```python
from build123d import *

# Parameters (mm, degrees)
SKETCH1_W            = 308.08168
SKETCH1_H            = 3.175
BOSS_EXTRUDE1_DEPTH  = 267.83
SKETCH3_W            = 267.83
SKETCH3_H            = 3.175
BOSS_EXTRUDE3_DEPTH  = 3.175
SKETCH4_W            = 50.8889
SKETCH4_H            = 3.175
BOSS_EXTRUDE4_DEPTH  = 267.83
CUT_EXTRUDE1_DEPTH   = 340.191055801
SKETCH17_W           = 267.83
SKETCH17_H           = 3.175
BOSS_EXTRUDE5_DEPTH  = 3.175
CUT_EXTRUDE3_DEPTH   = 340.191055801
SKETCH25_R           = 3.175
CUT_EXTRUDE8_DEPTH   = 3.175
SKETCH27_R           = 5
CUT_EXTRUDE9_DEPTH   = 340.191055801
SKETCH31_R           = 1.5875
CUT_EXTRUDE10_DEPTH  = 340.191055801
LPATTERN1_COUNT      = 3
LPATTERN1_PITCH      = 58
M4_CLEARANCE_HOLE1_D = 4.8
SKETCH36_W           = 57.15
SKETCH36_H           = 3.175
SKETCH36_W_2         = 26.9875
BOSS_EXTRUDE6_DEPTH  = 3.175
SKETCH37_W           = 3.175
SKETCH37_H           = 124.4419914
CUT_EXTRUDE11_DEPTH  = 340.191055801
SKETCH38_W           = 3.175
SKETCH38_H           = 146.0243
CUT_EXTRUDE12_DEPTH  = 340.191055801
SKETCH39_W           = 6.35
SKETCH39_H           = 9.525
CUT_EXTRUDE13_DEPTH  = 340.191055801


with BuildPart() as part:
    # Sketch1 → Boss-Extrude1 (new body)
    with BuildSketch(Plane.XY):
        Rectangle(SKETCH1_W, SKETCH1_H)
    extrude(amount=BOSS_EXTRUDE1_DEPTH)

    # Sketch3 → Boss-Extrude3 (add)
    with BuildSketch(Plane(origin=(154.04084, 0, 0), x_dir=(0, 0, -1), z_dir=(1, 0, 0))):
        with Locations((-133.915, 0)):
            Rectangle(SKETCH3_W, SKETCH3_H)
    extrude(amount=BOSS_EXTRUDE3_DEPTH)

    # Sketch4 → Boss-Extrude4 (add)
    with BuildSketch(Plane.XY.offset(267.83)):
        with Locations((182.66029, 0)):
            Rectangle(SKETCH4_W, SKETCH4_H)
    extrude(amount=-BOSS_EXTRUDE4_DEPTH)

    # Sketch6 → Cut-Extrude1 (cut, through all)
    with BuildSketch(Plane(origin=(0, 1.5875, 0), x_dir=(1, 0, 0), z_dir=(0, 1, 0))):
        Polygon((208.10474, -240.606362049), (106.50474, -267.83), (208.10474, -267.83), align=None)
    extrude(amount=-CUT_EXTRUDE1_DEPTH, mode=Mode.SUBTRACT)

    # Sketch17 → Boss-Extrude5 (add)
    with BuildSketch(Plane.ZY.offset(154.04084)):
        with Locations((133.915, 0)):
            Rectangle(SKETCH17_W, SKETCH17_H)
    extrude(amount=BOSS_EXTRUDE5_DEPTH)

    # Sketch11 → Cut-Extrude3 (cut, through all)
    with BuildSketch(Plane.XZ.offset(1.5875)):
        Polygon((-157.21584, 241.2743), (-84.254653892, 267.83), (-157.21584, 267.83), align=None)
    extrude(amount=-CUT_EXTRUDE3_DEPTH, mode=Mode.SUBTRACT)

    # Sketch25 → Cut-Extrude8 (cut)
    with BuildSketch(Plane.XZ.offset(1.5875)):
        with Locations(Location((-115.322188641, 247.921359373, 0), (0, 0, 270))):
            Circle(SKETCH25_R)
        with Locations(Location((-50.97526, 258.94, 0), (0, 0, 270))):
            Circle(SKETCH25_R)
        with Locations(Location((11.25474, 258.94, 0), (0, 0, 270))):
            Circle(SKETCH25_R)
        with Locations(Location((73.48474, 258.94, 0), (0, 0, 270))):
            Circle(SKETCH25_R)
        with Locations(Location((172.54474, 242.09298883, 0), (0, 0, 270))):
            Circle(SKETCH25_R)
        with Locations(Location((131.90474, 252.982444011, 0), (0, 0, 270))):
            Circle(SKETCH25_R)
    extrude(amount=-CUT_EXTRUDE8_DEPTH, mode=Mode.SUBTRACT)

    # Sketch27 → Cut-Extrude9 (cut, through all)
    with BuildSketch(Plane.XZ.offset(1.5875)):
        with Locations(Location((172.48674, 137.774823778, 0), (0, 0, 270))):
            Circle(SKETCH27_R)
        with Locations(Location((183.48674, 137.774823778, 0), (0, 0, 270))):
            Circle(SKETCH27_R)
        with Locations(Location((194.48674, 137.774823778, 0), (0, 0, 270))):
            Circle(SKETCH27_R)
        with Locations(Location((194.48674, 126.774823778, 0), (0, 0, 270))):
            Circle(SKETCH27_R)
        with Locations(Location((194.48674, 115.774823778, 0), (0, 0, 270))):
            Circle(SKETCH27_R)
        with Locations(Location((183.48674, 126.774823778, 0), (0, 0, 270))):
            Circle(SKETCH27_R)
        with Locations(Location((183.48674, 115.774823778, 0), (0, 0, 270))):
            Circle(SKETCH27_R)
        with Locations(Location((172.48674, 115.774823778, 0), (0, 0, 270))):
            Circle(SKETCH27_R)
        with Locations(Location((172.48674, 126.774823778, 0), (0, 0, 270))):
            Circle(SKETCH27_R)
        with Locations(Location((194.48674, 71.774823778, 0), (0, 0, 270))):
            Circle(SKETCH27_R)
        with Locations(Location((194.48674, 60.774823778, 0), (0, 0, 270))):
            Circle(SKETCH27_R)
        with Locations(Location((194.48674, 49.774823778, 0), (0, 0, 270))):
            Circle(SKETCH27_R)
        with Locations(Location((183.48674, 71.774823778, 0), (0, 0, 270))):
            Circle(SKETCH27_R)
        with Locations(Location((183.48674, 60.774823778, 0), (0, 0, 270))):
            Circle(SKETCH27_R)
        with Locations(Location((183.48674, 49.774823778, 0), (0, 0, 270))):
            Circle(SKETCH27_R)
        with Locations(Location((172.48674, 49.774823778, 0), (0, 0, 270))):
            Circle(SKETCH27_R)
        with Locations(Location((172.48674, 60.774823778, 0), (0, 0, 270))):
            Circle(SKETCH27_R)
        with Locations(Location((172.48674, 71.774823778, 0), (0, 0, 270))):
            Circle(SKETCH27_R)
    extrude(amount=-CUT_EXTRUDE9_DEPTH, mode=Mode.SUBTRACT)

    # Sketch31 → Cut-Extrude10 (cut, symmetric)
    with BuildSketch(Plane.XZ.offset(1.5875)):
        with Locations(Location((183.48674, 151.774823778, 0), (0, 0, 270))):
            Circle(SKETCH31_R)
    cut_extrude10 = extrude(amount=CUT_EXTRUDE10_DEPTH, both=True, mode=Mode.SUBTRACT)

    # LPattern1: Cut-Extrude10 ×3
    with Locations(*[(0, 0, -i * LPATTERN1_PITCH) for i in range(1, LPATTERN1_COUNT)]):
        add(cut_extrude10, mode=Mode.SUBTRACT)

    # M4 Clearance Hole1 (through all)
    with Locations(Plane.XZ.offset(1.5875)):
        with Locations((180.96500002, 176.776), (-97.77095, 213.2849914), (3.82905, 213.2849914), (105.42905, 213.2849914)):
            Hole(M4_CLEARANCE_HOLE1_D / 2)

    # Sketch36 → Boss-Extrude6 (add)
    with BuildSketch(Plane(origin=(0, 0, 0), x_dir=(-1, 0, 0), z_dir=(0, 0, -1))):
        Rectangle(SKETCH36_W, SKETCH36_H)
        with Locations((-182.66100002, 0)):
            Rectangle(SKETCH36_W_2, SKETCH36_H)
    extrude(amount=BOSS_EXTRUDE6_DEPTH)

    # Sketch37 → Cut-Extrude11 (cut, through all)
    with BuildSketch(Plane.XZ.offset(1.5875)):
        with Locations((155.62850002, 62.2209957)):
            Rectangle(SKETCH37_W, SKETCH37_H)
    extrude(amount=-CUT_EXTRUDE11_DEPTH, mode=Mode.SUBTRACT)

    # Sketch38 → Cut-Extrude12 (cut, through all)
    with BuildSketch(Plane.XZ.offset(1.5875)):
        with Locations((-155.62834, 73.01215)):
            Rectangle(SKETCH38_W, SKETCH38_H)
    extrude(amount=-CUT_EXTRUDE12_DEPTH, mode=Mode.SUBTRACT)

    # Sketch39 → Cut-Extrude13 (cut, through all)
    with BuildSketch(Plane.XZ.offset(1.5875)):
        with Locations((204.92974, 93.774823778)):
            Rectangle(SKETCH39_W, SKETCH39_H)
        with Locations((204.92974, 201.724823778)):
            Rectangle(SKETCH39_W, SKETCH39_H)
    extrude(amount=-CUT_EXTRUDE13_DEPTH, mode=Mode.SUBTRACT)


solid = part.part
```
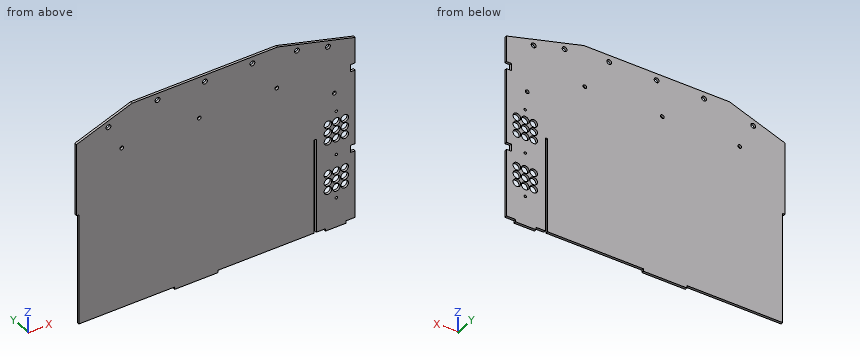
Can you work these out from the model? Positions are in its coordinate system, mm. Coordinates: 2 decimals unless noted, no trailing zeros. Loops run counter-clockwise (first coordinate to the right, second up) from the corner with the lowest first, then second, coordinate; pieces in that order, holes last.
Item 1: Suppose I cut it at B-B (x = 163.5). Please give me the cut outline in (y, z).
Answers below:
outline: (-1.59, 0) - (1.59, 0) - (1.59, 252.56) - (-1.59, 252.56) - close
Item 2: I'm going to push flat-ended pins straight in: pin 1 (9 mm diameter, centred on x = 194.49, z = 71.77, fed in from -Y); pin 2 (1 mm diameter, centred on x = 204.5, y = 0, fed in from -Z); pin 3 (1 mm diameter, centred on y = 0.5, z = 42.5, fed in from -X). Where does each tip first touch, or does it pass through?
Answers below:
pin 1: passes through
pin 2: stops at z = 0
pin 3: stops at x = -154.04
Item 3: Please list where these lines run through material, in increasing order: L1, parallel to X at y = -0.6, z = 49.5; L2, parallel to X at y = -1, z = 138.5; L3, parallel to X at y = 0.5, z = 110.5.
Answers below:
L1: x = -154.04 to 154.04, 157.22 to 167.49, 177.48 to 178.49, 188.48 to 189.49, 199.48 to 208.1
L2: x = -154.04 to 167.54, 177.43 to 178.54, 188.43 to 189.54, 199.43 to 208.1
L3: x = -154.04 to 154.04, 157.22 to 208.1
Item 4: Suppose I cut it at A-A (y = 0.4). State how many separate pieces and enclosed holes the cut face has, then the cut area to 3 significant figures.
Answers below:
separate pieces: 1
enclosed holes: 31
area: 93,100 mm2
